Autodesk Inventor part; units mm, degrees
ref_plane "YZ Plane" through (0, 0, 0) normal (1, 0, 0) x (0, 1, 0)
ref_plane "XZ Plane" through (0, 0, 0) normal (0, 1, 0) x (-1, 0, 0)
ref_plane "XY Plane" through (0, 0, 0) normal (0, 0, 1) x (1, 0, 0)
sketch "Schizzo1" plane through (0, 0, 0) normal (0, 0, 1) x (1, 0, 0)
  line L0 (4, 17) -> (0, 17) construction
  line L1 (0, 17) -> (0, 95) construction
  line L2 (0, 95) -> (4, 95) construction
  line L3 (4, 95) -> (4, 17) construction
  line L4 (4, -4) -> (4, -24) construction
  line L5 (4, -24) -> (0, -24) construction
  line L6 (0, -24) -> (0, -4) construction
  line L7 (0, 0) -> (0, 11) construction
  line L8 (0, 11) -> (4, 11) construction
  line L9 (4, 11) -> (4, 0) construction
  line L10 (-161, -24) -> (-161, 95)
  line L11 (-161, 95) -> (4, 95)
  line L12 (4, 95) -> (4, -24)
  line L13 (-133, -24) -> (-161, -24)
  arc A0 (-133, -24) -> (-128, -19) centre (-133, -19) ccw
  arc A1 (-123, -14) -> (-128, -19) centre (-123, -19) ccw
  line L14 (-100, -14) -> (-123, -14)
  arc A2 (-95, -19) -> (-100, -14) centre (-100, -19) ccw
  arc A3 (-95, -19) -> (-90, -24) centre (-90, -19) ccw
  line L15 (-67, -24) -> (-90, -24)
  arc A4 (-67, -24) -> (-62, -19) centre (-67, -19) ccw
  arc A5 (-57, -14) -> (-62, -19) centre (-57, -19) ccw
  line L16 (-34, -14) -> (-57, -14)
  arc A6 (-29, -19) -> (-34, -14) centre (-34, -19) ccw
  arc A7 (-29, -19) -> (-24, -24) centre (-24, -19) ccw
  line L17 (4, -24) -> (-24, -24)
  line L18 (-117, 13) -> (-37, 13) construction
  line L19 (-117, 3) -> (-37, 3)
  line L20 (-37, 23) -> (-117, 23)
  arc A8 (-117, 23) -> (-117, 3) centre (-117, 13) ccw
  arc A9 (-37, 3) -> (-37, 23) centre (-37, 13) ccw
  line L21 (-161, -4) -> (-150, -4)
  line L22 (-150, 0) -> (-150, -4)
  line L23 (-139, -4) -> (-128, -4)
  line L24 (-128, 0) -> (-128, -4)
  line L25 (-139, 0) -> (-128, 0)
  line L26 (-139, 0) -> (-139, -4)
  line L27 (-117, -4) -> (-106, -4)
  line L28 (-106, 0) -> (-106, -4)
  line L29 (-117, 0) -> (-106, 0)
  line L30 (-117, 0) -> (-117, -4)
  line L31 (-95, -4) -> (-84, -4)
  line L32 (-84, 0) -> (-84, -4)
  line L33 (-95, 0) -> (-84, 0)
  line L34 (-95, 0) -> (-95, -4)
  line L35 (-73, -4) -> (-62, -4)
  line L36 (-62, 0) -> (-62, -4)
  line L37 (-73, 0) -> (-62, 0)
  line L38 (-73, 0) -> (-73, -4)
  line L39 (-51, -4) -> (-40, -4)
  line L40 (-40, 0) -> (-40, -4)
  line L41 (-51, 0) -> (-40, 0)
  line L42 (-51, 0) -> (-51, -4)
  line L43 (-29, -4) -> (-18, -4)
  line L44 (-18, 0) -> (-18, -4)
  line L45 (-29, 0) -> (-18, 0)
  line L46 (-29, 0) -> (-29, -4)
  line L47 (-7, -4) -> (4, -4)
  line L48 (4, 0) -> (4, -4)
  line L49 (-7, 0) -> (4, 0)
  line L50 (-7, 0) -> (-7, -4)
  line L51 (-161, 0) -> (-150, 0)
  line L52 (-161, 0) -> (-161, -4)
  point P0 (-77, 13)
  dimension "d0" = 80
extrude "Estrusione1" add sketch "Schizzo1" along normal blind 4 contours L10 L21 L22 L51 L11 L12 L49 L50 L47 L17 A7 A6 L16 A5 A4 L15 A3 A2 L14 A1 A0 L13
sketch "Schizzo2" plane through (0, 0, 4) normal (0, 0, 1) x (1, 0, 0)
  line L0 (0, 76) -> (4, 76)
  line L1 (4, 76) -> (4, 66.5)
  line L2 (4, 66.5) -> (0, 66.5)
  line L3 (0, 66.5) -> (0, 76)
  line L4 (4, 85.5) -> (0, 85.5)
  line L5 (0, 85.5) -> (0, 95)
  line L6 (0, 95) -> (4, 95)
  line L7 (4, 95) -> (4, 85.5)
  line L8 (0, 38) -> (4, 38)
  line L9 (4, 38) -> (4, 28.5)
  line L10 (4, 28.5) -> (0, 28.5)
  line L11 (0, 28.5) -> (0, 38)
  line L12 (4, 47.5) -> (0, 47.5)
  line L13 (0, 47.5) -> (0, 57)
  line L14 (0, 57) -> (4, 57)
  line L15 (4, 57) -> (4, 47.5)
  line L16 (4, 9.5) -> (0, 9.5)
  line L17 (0, 9.5) -> (0, 19)
  line L18 (0, 19) -> (4, 19)
  line L19 (4, 19) -> (4, 9.5)
  point P0 (0, 0)
extrude "Estrusione2" cut sketch "Schizzo2" against normal blind 4
fillet "Raccordo1" radius 15 1 edges at (-161, 95, 2)
fillet "Raccordo2" radius 10 1 edges at (-161, -24, 2)
sketch "Schizzo3" plane through (0, 0, 4) normal (0, 0, 1) x (1, 0, 0)
  line L0 (-146.15, 0) -> (-142.85, 0)
  line L1 (-14.15, 0) -> (-10.85, 0)
  line L2 (-144.5, 0) -> (-144.5, 10) construction
  circle A0 centre (-144.5, 10) radius 1.65
  line L3 (-12.5, 0) -> (-12.5, 10) construction
  circle A1 centre (-12.5, 10) radius 1.65
  line L4 (0, 79.1) -> (0, 82.4) construction
  line L5 (0, -15.65) -> (0, -12.35) construction
  line L6 (0, -14) -> (-7, -14) construction
  line L7 (0, 80.75) -> (-7, 80.75) construction
  circle A2 centre (-7, 80.75) radius 1.65
  circle A3 centre (-7, -14) radius 1.65
  point P0 (0, 0)
  dimension "d7" = 10
  dimension "d8" = 3.3
  dimension "d9" = 10
  dimension "d10" = 3.3
  dimension "d13" = 7
  dimension "d14" = 7
  dimension "d15" = 3.3
  dimension "d16" = 3.3
extrude "Estrusione3" cut sketch "Schizzo3" against normal blind 4
properties part number "LatoPy"
Work out the finished part from the listing and answer in its coordinate system (mm). A direction names the side the tool comes from. Coordinates: 2 decimals unless noted, no trailing zeros. Loops run counter-clockwise (first coordinate to the right, second up) from the corner with the lowest first, then second, coordinate; pieces in that order, holes last. Notation, with made-up numbers: M 72.5,-5 L 118.5,-5 A24 ccw 118.5,29 Z; hole C 31,-20 d8. An arc over 180 degrees is marked long. Use CSV: the item, a comma, the result in double quotes. Start each with the question number.
(1) Find section B-B, the plane x = -12.5. Give the vertices of the cut face in (y, z), then the cut area to 3 significant figures.
(2) Find section C-C, the plane z = 1.95. State how many separate pieces and enclosed holes the cut face has, then the cut area to 3 significant figures.
(3) For a pull along X with two mould halves and no side action, classify faces 1 (the face through (-134, -4, 2)), 2 (the face through (-68, -4, 2)), 3 (the face through (-74, 95, 2)), 4 (the face through (4, 62, 2)) as +X half, -X half, draft (parallel to the pull), parting line (faces both ways), or undercut.
(4) Given pin 1 Ø1.2 at (y, z) = (-2, 2.5) entering from +X; pin 2 Ø2 at (y, z) = (32.5, 1.5) entering from +X, each flat-ended and moving along its own axis, determine where each tip first touches the part or whether it passes through.
(5) For faces 5 (the face through (2, 76, 2)), 6 (the face through (-46, -4, 2)), 7 (the face through (-156, -4, 2)), 8 (the face through (4, 43, 2)), determine the directions among +Z, -Z, +X, -X, +Y, -Y from which every point of the face is accessible in a straight line to the end or side of a thin tool.
(6) Consider line 1 (Y direction, x = -114.5, z = 0.75); line 2 (Y direction, x = -144.5, z = 2.35); line 3 (Y direction, x = -82.5, z = 0.3). Determine where each line is inside the solid, lowest interval first.
(7) Find section A-A, the plane x = -55. Give the vertices of the cut face in (y, z), then the cut area to 3 significant figures.
Recorded:
1,outline,"M -24,0 L 8.35,0 L 8.35,4 L -24,4 Z; M 11.65,0 L 95,0 L 95,4 L 11.65,4 Z"
1,area,"463 mm^2"
2,separate pieces,"1"
2,enclosed holes,"11"
2,area,"16,400 mm^2"
3,face 1,"undercut"
3,face 2,"undercut"
3,face 3,"draft"
3,face 4,"+X half"
4,pin 1,"stops at x = -7"
4,pin 2,"stops at x = 0"
5,face 5,"+Z, -Z, +X"
5,face 6,"+Z, -Z"
5,face 7,"+Z, -Z, -X"
5,face 8,"+Z, -Z, +X, +Y, -Y"
6,line 1,"y = -14 to -4, 0 to 3, 23 to 95"
6,line 2,"y = -24 to 8.35, 11.65 to 95"
6,line 3,"y = -24 to 3, 23 to 95"
7,outline,"M -14,0 L 3,0 L 3,4 L -14,4 Z; M 23,0 L 95,0 L 95,4 L 23,4 Z"
7,area,"356 mm^2"
